Input: part model. Units: mm. Frame: model coordinates. Face numbers are marked on the shaded views. A direction names the side the tool comes from. Give positions to 0.01 mm unless a question says otherwise; leave off trailing zeros. Order: outer loops, then holes, each group sorted by start corner. A loop starts at its lowest first (then second) coordinate and runs counter-clockwise, first axis right, second up. Notation, with made-up numbers: M 65.5,-24 L 88.5,-24 A13 cw 88.5,0 Z; hole C -18,-33 d11. An arc over 180 degrees is marked long. Use a Markdown table: item, result.
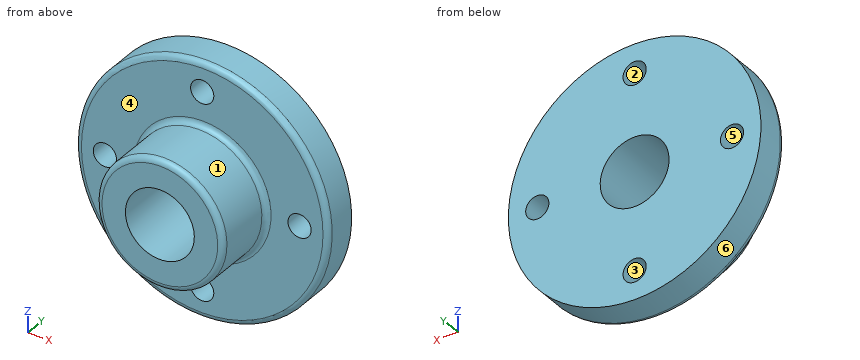
from build123d import *

# Parameters (mm, degrees)
F2_R            = 6.4164417579
F3_DEPTH        = 19.051
F3_COPIES_COUNT = 4
F4_R            = 3.048


# Not quite as in the source:
# - a pattern or mirror of a feature is missing from the dataset's text; its kind, count and spacing are read off the source's solid


with BuildPart() as f1:
    # F0 (on Right) → F1 (revolve)
    with BuildSketch(Plane.YZ):
        Polygon((-53.848, 19.05), (0, 19.05), (0, 69.85), (-19.05, 69.85), (-19.05, 35.052), (-53.848, 35.052), align=None)
    revolve(axis=Axis((0, -58.1718310714, 0), (0, -1, 0)))

    # F2 (on face) → F3 (cut, through all)
    with BuildSketch(Plane.XZ.offset(19.05)):
        with Locations((-53.848, 0)):
            Circle(F2_R)
    f3 = extrude(amount=-F3_DEPTH, mode=Mode.SUBTRACT)

    # F3_copies: F3 ×4 about axis
    f3_copies_axis = Axis((0, 0, 0), (0, 1, 0))
    for i in range(1, F3_COPIES_COUNT):
        add(f3.rotate(f3_copies_axis, i * 360 / F3_COPIES_COUNT), mode=Mode.SUBTRACT)

    # F4
    f4_edges = [f1.edges().sort_by_distance(p)[0] for p in [
        (0, -53.848, -35.052),
        (0, -19.05, -35.052),
        (0, -19.05, -69.85),
    ]]
    fillet(f4_edges, radius=F4_R)


solid = f1.part
1) Cut plane D-D on y = -10.5. Return loops of the section in (x, z).
Response values:
| item | result |
|---|---|
| outline | C 0,0 d139.7; hole C -53.85,0 d12.83; hole C 0,0 d38.1; hole C 0,-53.85 d12.83; hole C 0,53.85 d12.83; hole C 53.85,0 d12.83 |
2) Cut plane C-C on y = -28.5. Return loops of the section in (x, z), and give its area (3 significant figures).
Response values:
| item | result |
|---|---|
| outline | C 0,0 d70.1; hole C 0,0 d38.1 |
| area | 2,720 mm² |
3) Reachability of the marked faces 1 and 2 from +Z, -Z, +X, -X, +Y, -Y: full face, straight path, thin tool, end or side. Return the list, or none.
Response values:
| item | result |
|---|---|
| face 1 | -Y |
| face 2 | +Y, -Y |
4) Cut plane A-A on x = 0. Return loops of the section in (y, z).
Response values:
| item | result |
|---|---|
| outline | M -53.85,-32 A3.05 ccw -50.8,-35.05 L -22.1,-35.05 A3.05 cw -19.05,-38.1 L -19.05,-47.43 L 0,-47.43 L 0,-19.05 L -53.85,-19.05 Z; M -53.85,19.05 L 0,19.05 L 0,47.43 L -19.05,47.43 L -19.05,38.1 A3.05 cw -22.1,35.05 L -50.8,35.05 A3.05 ccw -53.85,32 Z; M -19.05,-66.8 A3.05 ccw -16,-69.85 L 0,-69.85 L 0,-60.26 L -19.05,-60.26 Z; M -19.05,60.26 L 0,60.26 L 0,69.85 L -16,69.85 A3.05 ccw -19.05,66.8 Z |
5) Material intervals for line 1 (Z direction, x = -2, y = -34); line 2 (Z direction, x = -6, y = -21); line 3 (X direction, y = -11.5, z = -56), sorted ascending. Write a range as from..to.
Response values:
| item | result |
|---|---|
| line 1 | z = -34.99..-18.94, 18.94..34.99 |
| line 2 | z = -34.74..-18.08, 18.08..34.74 |
| line 3 | x = -41.75..-6.04, 6.04..41.75 |
6) First-contact query: pin 1 Ø12 at (y, z) = (-18.5, 34) entering from -X; pin 2 Ø4 at (y, z) = (-27, 19) entering from +X; pin 3 Ø5 at (x, y) = (18, -35) entering from +Z; pin 4 Ø10.5 at (x, z) = (-53.848, 0) entering from +Y. Flat tips, straight axial feed; report the tip coordinate or a pass-through.
Response values:
| item | result |
|---|---|
| pin 1 | stops at x = -63.8 |
| pin 2 | stops at x = 30.65 |
| pin 3 | stops at z = 31.44 |
| pin 4 | passes through |
7) Cut plane B-B on z = 0. Return loops of the section in (x, y).
Response values:
| item | result |
|---|---|
| outline | M -69.85,-16 A3.05 ccw -66.8,-19.05 L -60.26,-19.05 L -60.26,0 L -69.85,0 Z; M -47.43,-19.05 L -38.1,-19.05 A3.05 cw -35.05,-22.1 L -35.05,-50.8 A3.05 ccw -32,-53.85 L -19.05,-53.85 L -19.05,0 L -47.43,0 Z; M 19.05,-53.85 L 32,-53.85 A3.05 ccw 35.05,-50.8 L 35.05,-22.1 A3.05 cw 38.1,-19.05 L 47.43,-19.05 L 47.43,0 L 19.05,0 Z; M 60.26,-19.05 L 66.8,-19.05 A3.05 ccw 69.85,-16 L 69.85,0 L 60.26,0 Z |
8) Mould query, pull axis X, two halves, no side actions, for the marked faces 3, 4, 5 and 6. Classes: released by +X, released by -X, zero draft, split by the parting line, or undercut.
Response values:
| item | result |
|---|---|
| face 3 | undercut |
| face 4 | zero draft |
| face 5 | undercut |
| face 6 | split by the parting line |
